```python
from build123d import *

# Parameters (mm, degrees)
F0_R     = 1.1938
F1_DEPTH = 1.6002
F2_D     = 3.175
F3_R     = 5.08


with BuildPart() as f1:
    # F0 (on Top) → F1 (new body)
    with BuildSketch(Plane.XY):
        Polygon((-94.253136, -22.86), (55.606864, -22.86), (60.686864, -22.86), (60.686864, 33.02), (55.606864, 33.02), (-94.253136, 33.02), (-99.333136, 33.02), (-99.333136, -22.86), align=None)
        with Locations((53.066864, -17.78)):
            Circle(F0_R, mode=Mode.SUBTRACT)
        with BuildLine():
            ThreePointArc((55.606864, -18.9738), (54.413064, -17.78), (55.606864, -16.5862))
            ThreePointArc((55.606864, -16.5862), (56.451008, -16.935856), (56.800664, -17.78))
            ThreePointArc((56.800664, -17.78), (56.451008, -18.624144), (55.606864, -18.9738))
        make_face(mode=Mode.SUBTRACT)
        with Locations((53.066864, -15.24)):
            Circle(F0_R, mode=Mode.SUBTRACT)
        with BuildLine():
            ThreePointArc((55.606864, -16.4338), (54.413064, -15.24), (55.606864, -14.0462))
            ThreePointArc((55.606864, -14.0462), (56.451008, -14.395856), (56.800664, -15.24))
            ThreePointArc((56.800664, -15.24), (56.451008, -16.084144), (55.606864, -16.4338))
        make_face(mode=Mode.SUBTRACT)
        with Locations((53.066864, -10.16)):
            Circle(F0_R, mode=Mode.SUBTRACT)
        with BuildLine():
            ThreePointArc((55.606864, -11.3538), (54.413064, -10.16), (55.606864, -8.9662))
            ThreePointArc((55.606864, -8.9662), (56.451008, -9.315856), (56.800664, -10.16))
            ThreePointArc((56.800664, -10.16), (56.451008, -11.004144), (55.606864, -11.3538))
        make_face(mode=Mode.SUBTRACT)
        with Locations((53.066864, -7.62)):
            Circle(F0_R, mode=Mode.SUBTRACT)
        with BuildLine():
            ThreePointArc((56.800664, -7.62), (56.451008, -8.464144), (55.606864, -8.8138))
            ThreePointArc((55.606864, -8.8138), (54.413064, -7.62), (55.606864, -6.4262))
            ThreePointArc((55.606864, -6.4262), (56.451008, -6.775856), (56.800664, -7.62))
        make_face(mode=Mode.SUBTRACT)
        with Locations((53.066864, -5.08)):
            Circle(F0_R, mode=Mode.SUBTRACT)
        with BuildLine():
            ThreePointArc((56.800664, -5.08), (56.451008, -5.924144), (55.606864, -6.2738))
            ThreePointArc((55.606864, -6.2738), (54.413064, -5.08), (55.606864, -3.8862))
            ThreePointArc((55.606864, -3.8862), (56.451008, -4.235856), (56.800664, -5.08))
        make_face(mode=Mode.SUBTRACT)
        with Locations((53.066864, -2.54)):
            Circle(F0_R, mode=Mode.SUBTRACT)
        with BuildLine():
            ThreePointArc((56.800664, -2.54), (56.451008, -3.384144), (55.606864, -3.7338))
            ThreePointArc((55.606864, -3.7338), (54.413064, -2.54), (55.606864, -1.3462))
            ThreePointArc((55.606864, -1.3462), (56.451008, -1.695856), (56.800664, -2.54))
        make_face(mode=Mode.SUBTRACT)
        with Locations((53.066864, 0)):
            Circle(F0_R, mode=Mode.SUBTRACT)
        with BuildLine():
            ThreePointArc((56.800664, 0), (56.451008, -0.844144), (55.606864, -1.1938))
            ThreePointArc((55.606864, -1.1938), (54.413064, 0), (55.606864, 1.1938))
            ThreePointArc((55.606864, 1.1938), (56.451008, 0.844144), (56.800664, 0))
        make_face(mode=Mode.SUBTRACT)
        with Locations((50.526864, 10.16)):
            Circle(F0_R, mode=Mode.SUBTRACT)
        with Locations((53.066864, 10.16)):
            Circle(F0_R, mode=Mode.SUBTRACT)
        with BuildLine():
            ThreePointArc((56.800664, 10.16), (56.451008, 9.315856), (55.606864, 8.9662))
            ThreePointArc((55.606864, 8.9662), (54.413064, 10.16), (55.606864, 11.3538))
            ThreePointArc((55.606864, 11.3538), (56.451008, 11.004144), (56.800664, 10.16))
        make_face(mode=Mode.SUBTRACT)
        with Locations((50.526864, 12.7)):
            Circle(F0_R, mode=Mode.SUBTRACT)
        with Locations((50.526864, 15.24)):
            Circle(F0_R, mode=Mode.SUBTRACT)
        with Locations((53.066864, 12.7)):
            Circle(F0_R, mode=Mode.SUBTRACT)
        with BuildLine():
            ThreePointArc((56.800664, 12.7), (56.451008, 11.855856), (55.606864, 11.5062))
            ThreePointArc((55.606864, 11.5062), (54.413064, 12.7), (55.606864, 13.8938))
            ThreePointArc((55.606864, 13.8938), (56.451008, 13.544144), (56.800664, 12.7))
        make_face(mode=Mode.SUBTRACT)
        with Locations((53.066864, 15.24)):
            Circle(F0_R, mode=Mode.SUBTRACT)
        with BuildLine():
            ThreePointArc((56.800664, 15.24), (56.451008, 14.395856), (55.606864, 14.0462))
            ThreePointArc((55.606864, 14.0462), (54.413064, 15.24), (55.606864, 16.4338))
            ThreePointArc((55.606864, 16.4338), (56.451008, 16.084144), (56.800664, 15.24))
        make_face(mode=Mode.SUBTRACT)
        with Locations((50.526864, 17.78)):
            Circle(F0_R, mode=Mode.SUBTRACT)
        with Locations((53.066864, 17.78)):
            Circle(F0_R, mode=Mode.SUBTRACT)
        with BuildLine():
            ThreePointArc((56.800664, 17.78), (56.451008, 16.935856), (55.606864, 16.5862))
            ThreePointArc((55.606864, 16.5862), (54.413064, 17.78), (55.606864, 18.9738))
            ThreePointArc((55.606864, 18.9738), (56.451008, 18.624144), (56.800664, 17.78))
        make_face(mode=Mode.SUBTRACT)
        with Locations((50.526864, 20.32)):
            Circle(F0_R, mode=Mode.SUBTRACT)
        with Locations((53.066864, 20.32)):
            Circle(F0_R, mode=Mode.SUBTRACT)
        with BuildLine():
            ThreePointArc((56.800664, 20.32), (56.451008, 19.475856), (55.606864, 19.1262))
            ThreePointArc((55.606864, 19.1262), (54.413064, 20.32), (55.606864, 21.5138))
            ThreePointArc((55.606864, 21.5138), (56.451008, 21.164144), (56.800664, 20.32))
        make_face(mode=Mode.SUBTRACT)
        with Locations((50.526864, 25.4)):
            Circle(F0_R, mode=Mode.SUBTRACT)
        with Locations((53.066864, 25.4)):
            Circle(F0_R, mode=Mode.SUBTRACT)
        with BuildLine():
            ThreePointArc((56.800664, 25.4), (56.451008, 24.555856), (55.606864, 24.2062))
            ThreePointArc((55.606864, 24.2062), (54.413064, 25.4), (55.606864, 26.5938))
            ThreePointArc((55.606864, 26.5938), (56.451008, 26.244144), (56.800664, 25.4))
        make_face(mode=Mode.SUBTRACT)
        with Locations((50.526864, 27.94)):
            Circle(F0_R, mode=Mode.SUBTRACT)
        with Locations((53.066864, 27.94)):
            Circle(F0_R, mode=Mode.SUBTRACT)
        with BuildLine():
            ThreePointArc((56.800664, 27.94), (56.451008, 27.095856), (55.606864, 26.7462))
            ThreePointArc((55.606864, 26.7462), (54.76272, 28.784144), (56.800664, 27.94))
        make_face(mode=Mode.SUBTRACT)
    extrude(amount=-F1_DEPTH)

    # F2 (through all)
    with Locations(Plane.XY):
        with Locations((-94.253136, 5.08), (-19.323136, 5.08), (55.606864, 5.08)):
            Hole(F2_D / 2)

    # F3
    f3_edges = [f1.edges().sort_by_distance(p)[0] for p in [
        (60.686864, -22.86, -0.8001),
        (60.686864, 33.02, -0.8001),
        (-99.333136, -22.86, -0.8001),
        (-99.333136, 33.02, -0.8001),
    ]]
    fillet(f3_edges, radius=F3_R)


solid = f1.part
```
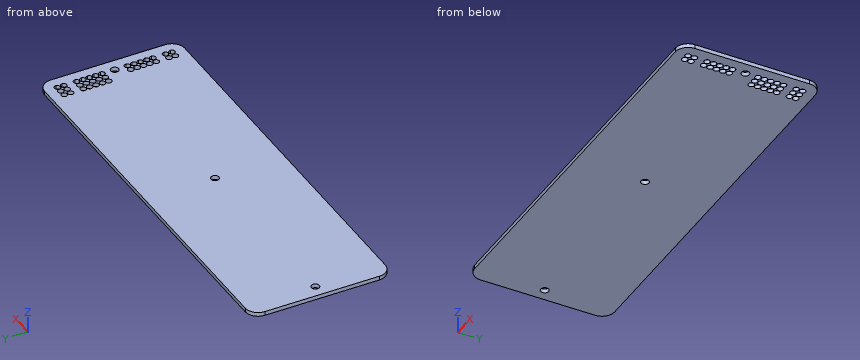
The model under review builds one solid part; all positions refer to its coordinate system, in mm. Round coordinates to 2 decimals unless told otherwise and drop trailing zeros. Write each loop counter-clockwise with the first axis right and the second up, starting at its lowest first coordinate (ties: lowest second). Pieces come first, ordered by that corner, then holes.
(1) We need section A-A on y = 5.08. Give the boundary of the cut face in (x, z).
(2) Wall thickness on L1, parallel to X at y = 6, z = -0.9; L2, parallel to X at y = -9.5, z = -0.3; L3, parallel to X at y = 13, z = -0.1: over which ranges is each line inside the solid? List them lowest first.
(3) We need section B-B on z = -1.35. Give the number of separate pieces and of enclosed holes in the cut face, and give its area (3 significant figures).
Findings below:
1. outline: (-99.33, -1.6) - (-95.84, -1.6) - (-95.84, 0) - (-99.33, 0) - close; (-92.67, -1.6) - (-20.91, -1.6) - (-20.91, 0) - (-92.67, 0) - close; (-17.74, -1.6) - (54.02, -1.6) - (54.02, 0) - (-17.74, 0) - close; (57.19, -1.6) - (60.69, -1.6) - (60.69, 0) - (57.19, 0) - close
2. L1: x = -99.33 to -95.55, -92.96 to -20.62, -18.03 to 54.31, 56.9 to 60.69
2. L2: x = -99.33 to 52.07, 54.06 to 54.61, 56.6 to 60.69
2. L3: x = -99.33 to 49.37, 51.68 to 51.91, 54.22 to 54.45, 56.76 to 60.69
3. separate pieces: 1
3. enclosed holes: 38
3. area: 8,740 mm2
